Job drawing, mm, ordinate dimensions from the low corner. One solid piece. Give positions to 0.01 mm unless a question says otherwise; leave off trailing zeros. Write each loop counter-clockwise with the first axis right and the second up, starting at its lowest first coordinate (ties: lowest second). Pieces come first, ordered by that corner, then holes. Notation, with made-up numbers: (54.25, 71.25) - (70.25, 71.25) arc R24 cw to (70.25, 95.25) - close; hole circle Ø4 at (-39, 66.25). An arc over 180 degrees is marked (long way). Answer as a JSON object with one key per item and string values.
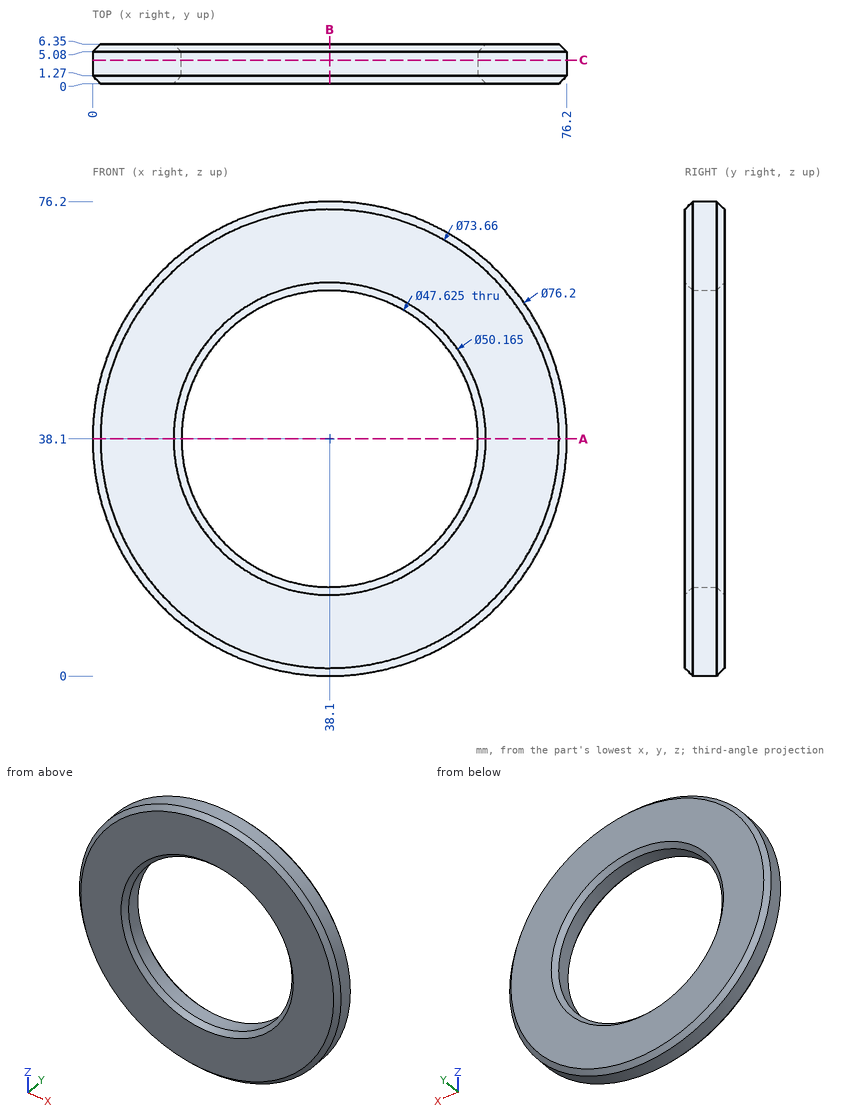
Item 1: Probe line 1 (Z direction, x = 38.1, y = 2.8); line 2 (Z direction, x = 53, y = 1); line 3 (X direction, y = 1.25, z = 56). List the from-to ranges inside material, lowest first. Write a range as from..to.
Entries:
{"line 1": "0..14.29, 61.91..76.2", "line 2": "3.33..19.18, 57.02..72.87", "line 3": "4.49..22.37, 53.83..71.71"}
Item 2: Cut at C-C (y = 3.75). Give the cut face in (x, z) (1 decimal).
Entries:
{"outline": "circle Ø76.2 at (38.1, 38.1); hole circle Ø47.6 at (38.1, 38.1)"}
Item 3: Cut at B-B (x = 38.1). Give the cut face in (y, z).
Entries:
{"outline": "(0, 1.27) - (1.27, 0) - (5.08, 0) - (6.35, 1.27) - (6.35, 13.02) - (5.08, 14.29) - (1.27, 14.29) - (0, 13.02) - close; (0, 63.18) - (1.27, 61.91) - (5.08, 61.91) - (6.35, 63.18) - (6.35, 74.93) - (5.08, 76.2) - (1.27, 76.2) - (0, 74.93) - close"}
Item 4: Flat gauge pins, fed straight in: P1, Ø2, axis at y = 5.5, z = 19.5, coming from the -X side; P2, Ø2, axis at x = 29.5, y = 4.5, coming from the -Z side; P3, Ø1, axis at y = 3.5, z = 65.5, coming from the -X side. Where does each tip first touch, or does it go through?
Entries:
{"P1": "x = 4.36", "P2": "z = 0.77", "P3": "x = 11.12"}
Item 5: Cut at A-A (z = 38.1). Give the cut face in (x, y).
Entries:
{"outline": "(0, 1.27) - (1.27, 0) - (13.02, 0) - (14.29, 1.27) - (14.29, 5.08) - (13.02, 6.35) - (1.27, 6.35) - (0, 5.08) - close; (61.91, 1.27) - (63.18, 0) - (74.93, 0) - (76.2, 1.27) - (76.2, 5.08) - (74.93, 6.35) - (63.18, 6.35) - (61.91, 5.08) - close"}
